Source: CAD feature listing. Evaluate the final solid. Frame: model axes, mm. Face numbers are marked on the shaded views. A direction names the side the tool comes from. Give positions to 0.01 mm unless a question says otherwise; leave off trailing zeros. Loops run counter-clockwise (first coordinate to the right, second up) from the corner with the lowest first, then second, coordinate; pieces in that order, holes last. Notation, with made-up numbers: (6, -10) -> (10, -10) arc R15 ccw to (10, 14) -> close; hole circle Ø3 at (12.25, 0.25). An arc over 180 degrees is marked (long way). Put each result on its own line as item: value.
```python
from build123d import *

# Parameters (mm, degrees)
F0_R     = 76.389164
F1_DEPTH = 519.66989
F2_W     = 274.323284
F2_H     = 235.549598
F3_DEPTH = 83.782351
F4_SIZE  = 101.6


with BuildPart() as f1:
    # F0 (on Front) → F1 (new body)
    with BuildSketch(Plane.XZ):
        Circle(F0_R)
    extrude(amount=-F1_DEPTH)

    # F2 (on Front) → F3 (join)
    with BuildSketch(Plane.XZ):
        Rectangle(F2_W, F2_H)
    extrude(amount=F3_DEPTH)

    # F4
    f4_edges = [f1.edges().sort_by_distance(p)[0] for p in [
        (137.161642, -41.891175, 117.774799),
        (-137.161642, -41.891175, 117.774799),
        (-137.161642, -41.891175, -117.774799),
        (137.161642, -41.891175, -117.774799),
    ]]
    chamfer(f4_edges, length=F4_SIZE)


solid = f1.part
```
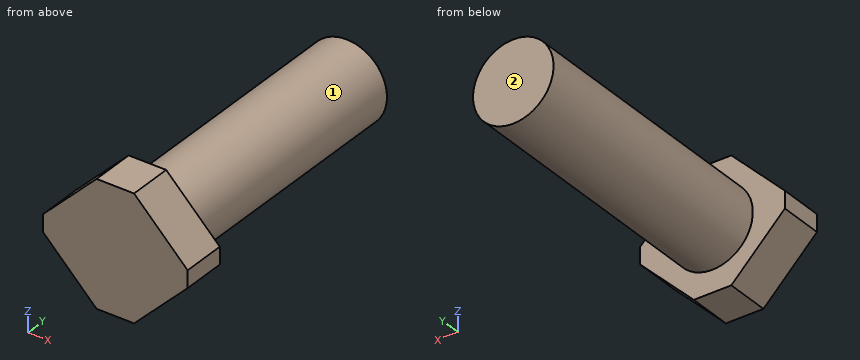
(1) Section A-A on x = 0. Return loops of the section in (y, z).
Calculated:
outline: (-83.78, -117.77) -> (0, -117.77) -> (0, -76.39) -> (519.67, -76.39) -> (519.67, 76.39) -> (0, 76.39) -> (0, 117.77) -> (-83.78, 117.77) -> close
(2) Section D-D on z = -86. Return loops of the section in (x, y), then the cut area to 3 significant figures.
Calculated:
outline: (-67.34, -83.78) -> (67.34, -83.78) -> (67.34, 0) -> (-67.34, 0) -> close
area: 11,300 mm²
(3) Reachability of the marked faces 1 and 2 from +Z, -Z, +X, -X, +Y, -Y: full face, straight path, thin tool, end or side. Return the list, or none.
Calculated:
face 1: +Y
face 2: +Z, -Z, +X, -X, +Y
(4) Section B-B on z = 0. Return loops of the section in (x, y).
Calculated:
outline: (-137.16, -83.78) -> (137.16, -83.78) -> (137.16, 0) -> (76.39, 0) -> (76.39, 519.67) -> (-76.39, 519.67) -> (-76.39, 0) -> (-137.16, 0) -> close
(5) Section C-C on y = 291. Return loops of the section in (x, z), then the cut area to 3 significant figures.
Calculated:
outline: circle Ø152.78 at (0, 0)
area: 18,300 mm²
(6) First-contact query: P1, Ø8, axis at y = 373.5, z = -53, coming from the +X side; P2, Ø4, axis at x = 76.5, z = -24, coming from the +Y side; P3, Ø1, axis at y = 39.5, z = 70.5, coming from the -X side. Flat tips, straight axial feed; report the tip coordinate or a pass-through.
Calculated:
P1: stops at x = 58.6
P2: stops at y = 0
P3: stops at x = -30.58
(7) Line query: probe 1 along Z at (x, y) = (3, 408.5); probe 2 along Y at (x, z) = (53, -59); probe 3 along Z at (x, y) = (-103, -33). Output: solid intervals per line, ascending. Write a range as from..to.
Calculated:
probe 1: z = -76.33..76.33
probe 2: y = -83.78..0
probe 3: z = -50.34..50.34
